Check sheet for the modelled part. Datum: model origin and axes. Units: mm. Coordinates: 2 decimals unless noted, no trailing zeros. Loops run counter-clockwise (first coordinate to the right, second up) from the corner with the lowest first, then second, coordinate; pieces in that order, holes last. Notation, with made-up numbers: (12.25, 77) -> (35.25, 77) arc R29 ccw to (35.25, 114) -> close; hole circle Ø2 at (19.5, 56.5). An arc over 180 degrees is marked (long way). Use CSV: the item, a comma, the result in double quotes.
```python
from build123d import *

# Parameters (mm, degrees)
SKETCH1_W           = 33
SKETCH1_H           = 39
SKETCH1_R           = 2.5
SKETCH1_R_2         = 3.5
BOSS_EXTRUDE1_DEPTH = 1.8
FILLET1_R           = 4
FILLET2_R           = 4
FILLET3_R           = 4
FILLET4_R           = 4


with BuildPart() as part:
    # Sketch1 → Boss-Extrude1 (new body)
    with BuildSketch(Plane(origin=(0, 0, 0), x_dir=(1, 0, 0), z_dir=(0, 1, 0))):
        Rectangle(SKETCH1_W, SKETCH1_H)
        with Locations(Location((12, -15, 0), (0, 0, 270))):
            Circle(SKETCH1_R, mode=Mode.SUBTRACT)
        with Locations(Location((12, 15, 0), (0, 0, 90))):
            Circle(SKETCH1_R, mode=Mode.SUBTRACT)
        with Locations(Location((-12, -15, 0), (0, 0, 90))):
            Circle(SKETCH1_R, mode=Mode.SUBTRACT)
        with Locations(Location((-12, 15, 0), (0, 0, 270))):
            Circle(SKETCH1_R, mode=Mode.SUBTRACT)
        with Locations(Location((0, 0, 0), (0, 0, 270))):
            Circle(SKETCH1_R_2, mode=Mode.SUBTRACT)
    extrude(amount=BOSS_EXTRUDE1_DEPTH)

    # Fillet1
    fillet1_edges = [part.edges().sort_by_distance(p)[0] for p in [
        (-16.5, 0.9, -19.5),
    ]]
    fillet(fillet1_edges, radius=FILLET1_R)

    # Fillet2
    fillet2_edges = [part.edges().sort_by_distance(p)[0] for p in [
        (16.5, 0.9, -19.5),
    ]]
    fillet(fillet2_edges, radius=FILLET2_R)

    # Fillet3
    fillet3_edges = [part.edges().sort_by_distance(p)[0] for p in [
        (16.5, 0.9, 19.5),
    ]]
    fillet(fillet3_edges, radius=FILLET3_R)

    # Fillet4
    fillet4_edges = [part.edges().sort_by_distance(p)[0] for p in [
        (-16.5, 0.9, 19.5),
    ]]
    fillet(fillet4_edges, radius=FILLET4_R)


solid = part.part
```
1) Draft check along Z on faces 1 (the flat face through (0, 1, 19.5)), 2 (the cylindrical face through (10.5, 0.9, 13)), 3 (the flat face through (0, 1, -19.5)), 4 (the cylindrical face through (13.5, 0.9, -13)). Enter one of: released by +Z, released by -Z, zero draft, split by the parting line, or undercut.
Answer below:
face 1,"released by +Z"
face 2,"undercut"
face 3,"released by -Z"
face 4,"undercut"
2) Thickness scan on line 1 along X through (y, z) = (1.35, -15); line 2 along X through (y, z) = (0.7, -16); line 3 along Z through (x, y) = (13.5, 0.75). Record the ranges inside material, lowest first. Write a range as from..to.
Answer below:
line 1,"x = -16.5..-14.5, -9.5..9.5, 14.5..16.5"
line 2,"x = -16.47..-14.29, -9.71..9.71, 14.29..16.47"
line 3,"z = -19.37..-17, -13..13, 17..19.37"
3) Cross-section at A-A on x = 0. Record the boundary of the cut face in (y, z).
Answer below:
outline,"(0, -19.5) -> (1.8, -19.5) -> (1.8, -3.5) -> (0, -3.5) -> close; (0, 3.5) -> (1.8, 3.5) -> (1.8, 19.5) -> (0, 19.5) -> close"
4) Cross-section at D-D on z = -13.5. Record the boundary of the cut face in (x, y).
Answer below:
outline,"(-16.5, 0) -> (-14, 0) -> (-14, 1.8) -> (-16.5, 1.8) -> close; (-10, 0) -> (10, 0) -> (10, 1.8) -> (-10, 1.8) -> close; (14, 0) -> (16.5, 0) -> (16.5, 1.8) -> (14, 1.8) -> close"
5) Cross-section at C-C on x = -12. Record the boundary of the cut face in (y, z), and give its area (3 significant figures).
Answer below:
outline,"(0, -19.5) -> (1.8, -19.5) -> (1.8, -17.5) -> (0, -17.5) -> close; (0, -12.5) -> (1.8, -12.5) -> (1.8, 12.5) -> (0, 12.5) -> close; (0, 17.5) -> (1.8, 17.5) -> (1.8, 19.5) -> (0, 19.5) -> close"
area,"52.2 mm²"
6) Cross-section at B-B on y = 1.2. Record the boundary of the cut face in (x, z).
Answer below:
outline,"(-16.5, -15.5) arc R4 ccw to (-12.5, -19.5) -> (12.5, -19.5) arc R4 ccw to (16.5, -15.5) -> (16.5, 15.5) arc R4 ccw to (12.5, 19.5) -> (-12.5, 19.5) arc R4 ccw to (-16.5, 15.5) -> close; hole circle Ø5 at (-12, -15); hole circle Ø5 at (-12, 15); hole circle Ø7 at (0, 0); hole circle Ø5 at (12, -15); hole circle Ø5 at (12, 15)"
